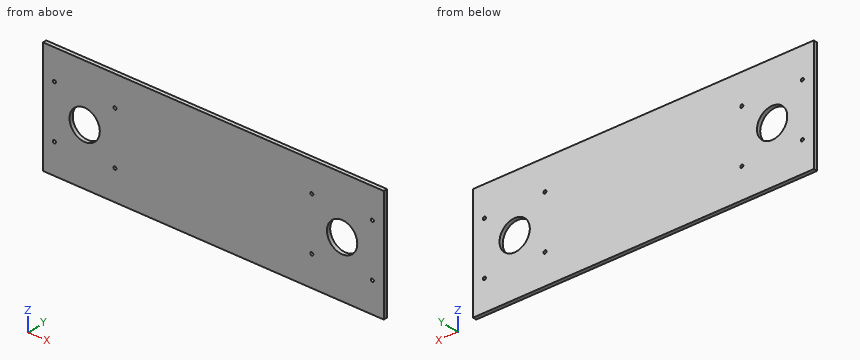
Autodesk Inventor part; units mm, degrees
ref_plane "YZ Plane" through (0, 0, 0) normal (1, 0, 0) x (0, 1, 0)
ref_plane "XZ Plane" through (0, 0, 0) normal (0, 1, 0) x (-1, 0, 0)
ref_plane "XY Plane" through (0, 0, 0) normal (0, 0, 1) x (1, 0, 0)
sketch "Sketch1" plane through (0, 0, 0) normal (0, 1, 0) x (-1, 0, 0)
  line L0 (225, 75) -> (-225, 75)
  line L1 (-225, 75) -> (-225, -75)
  line L2 (-225, -75) -> (225, -75)
  line L3 (225, -75) -> (225, 75)
  line L4 (225, 75) -> (-225, -75) construction
  line L5 (-225, 75) -> (225, -75) construction
  point P0 (0, 0)
  dimension "d0" = 450
  dimension "d1" = 150
extrude "Extrusion1" add sketch "Sketch1" along normal blind 5
sketch "Sketch2" plane through (0, 5, 0) normal (0, 1, 0) x (1, 0, 0)
  circle A0 centre (-210, -35) radius 2.05
  circle A1 centre (-130, 35) radius 2.05
  circle A2 centre (-130, -35) radius 2.05
  circle A3 centre (-210, 35) radius 2.05
  arc A4 (-190.5, 40) -> (-194.5, 44.899) centre (-195.5, 40) ccw
  line L0 (-190.5, 40) -> (-190.5, -20)
  line L1 (-190.5, -20) -> (-149.5, -20)
  line L2 (-149.5, -20) -> (-149.5, 56)
  line L3 (-180, 56) -> (-180, 75)
  line L4 (-180, 75) -> (-120, 75)
  line L5 (-120, 75) -> (-120, -75)
  line L6 (-120, -75) -> (-220, -75)
  line L7 (-220, -75) -> (-220, 75)
  line L8 (-220, 75) -> (-198.5, 75)
  line L9 (-198.5, 75) -> (-198.5, 49.798)
  arc A5 (-198.5, 49.798) -> (-194.5, 44.899) centre (-193.5, 49.798) ccw
  circle A6 centre (-210, 35) radius 2
  circle A7 centre (-210, -35) radius 2
  circle A8 centre (-130, -35) radius 2
  circle A9 centre (-130, 35) radius 2
  line L10 (-149.5, 56) -> (-180, 56)
  point P0 (0, 0)
  dimension "d4" = 4
  dimension "d5" = 4
  dimension "d6" = 4
  dimension "d7" = 4
extrude "Extrusion2" cut sketch "Sketch2" against normal blind 5 contours A6 | A7 | A8 | A9
mirror "Mirror1" about plane through (0, 0, 0) normal (1, 0, 0) of "Extrusion2"
sketch "Sketch4" plane through (0, 0, 0) normal (0, -1, 0) x (1, 0, 0)
  line L0 (62, 45) -> (62, 5)
  circle A0 centre (210, -35) radius 2
  circle A1 centre (130, -35) radius 2
  circle A2 centre (210, 35) radius 2
  circle A3 centre (130, 35) radius 2
  circle A4 centre (-130, 35) radius 2
  circle A5 centre (-210, 35) radius 2
  circle A6 centre (-130, -35) radius 2
  circle A7 centre (-210, -35) radius 2
  line L1 (225, 75) -> (225, -75)
  line L2 (-225, 75) -> (225, 75)
  line L3 (-225, -75) -> (-225, 75)
  line L4 (225, -75) -> (-225, -75)
  circle A8 centre (-170, 0) radius 20
  circle A9 centre (170, 0) radius 20
  point P0 (0, 0)
  dimension "d16" = 40
  dimension "d17" = 40
extrude "Extrusion4" cut sketch "Sketch4" against normal blind 5 contours A8 | A9
properties part number "acrylic_back"
Source: CAD feature listing. Evaluate the final solid. Frame: model axes, mm. Give positions to 0.01 mm unless a question says otherwise; leave off trailing zeros. Order: outer loops, then holes, each group sorted by start corner. A loop starts at its lowest first (then second) coordinate and runs counter-clockwise, first axis right, second up.
(1) Section query C-C (z = -5). Return the cut outline in (x, y).
(2) Section query B-B (y = 3.65). State how many separate pieces and enclosed holes the cut face has, plus the area to 3 significant figures.
(3) Contact query for a flat-ended pin moving along its axis: P1, Ø4.5, axis at x = 130, z = -35, coming from the -Y side. Output: stop coordinate, or through.
(4) Section query A-A (x = 170). Return the cut outline in (y, z).
(5) Material intervals for line 1 along Z through (x, y) = (-130, 2.2); line 2 along X through (y, z) = (3.85, -35); line 3 along X through (y, z) = (2.6, 6), sorted ascending.
Outcome:
1. outline: (-225, 0) - (-189.36, 0) - (-189.36, 5) - (-225, 5) - close; (-150.64, 0) - (150.64, 0) - (150.64, 5) - (-150.64, 5) - close; (189.36, 0) - (225, 0) - (225, 5) - (189.36, 5) - close
2. separate pieces: 1
2. enclosed holes: 10
2. area: 64,900 mm2
3. P1: stops at y = 0
4. outline: (0, -75) - (5, -75) - (5, -20) - (0, -20) - close; (0, 20) - (5, 20) - (5, 75) - (0, 75) - close
5. line 1: z = -75 to -37, -33 to 33, 37 to 75
5. line 2: x = -225 to -212, -208 to -132, -128 to 128, 132 to 208, 212 to 225
5. line 3: x = -225 to -189.08, -150.92 to 150.92, 189.08 to 225
